Design review of the part shown in the three views and the two pictorial views. Dimensions are in mm from the part's minimum x, y and z. A direction names the side the tool comes from. Coordinates: 2 decimals unless noted, no trailing zeros. Write each loop counter-clockwise with the first axis right and the second up, starting at its lowest first coordinate (ties: lowest second). Pieces come first, ordered by that corner, then holes. Notation, with made-up numbers: (0, -2.75) -> (6, -2.75) arc R17 ccw to (6, 19.25) -> close; hole circle Ø5 at (73, -33). An arc over 180 degrees is marked (long way). Answer in a Markdown table with one row per item. Add a question column.
Item 1: Take a section at A-A, the plane x = 67. Write out the cut boundary in (y, z).
Item 2: To check wall thickness, follow line 1 (Y direction, x = 63, z = 36.5); line 2 (Z direction, x = 106, y = 40); line 3 (Z direction, x = 150, y = 5.5) (1 decimal). State the ranges of each line that lie inside material, in increasing order.
Item 3: Take a section at D-D, the plane x = 111. Write out the cut boundary in (y, z).
Item 4: For the marked faces 1 and 2, list the 3-axis set-ups (+Z, -Z, +X, -X, +Y, -Y) from which the entire face can be reached by the end or side of a thin tool; tool diameter is ignored.
Item 5: Take a section at B-B, the plane z = 10. Write out the cut boundary in (x, y), and give its area (3 significant figures).
Item 6: Clearance check with flat-ended pins moving along their axes: P1, Ø3.5, axis at y = 30, z = 51.5, coming from the +X side; P2, Ø16, axis at x = 91.5, z = 15, coming from the +Y side; P3, Ø12, axis at x = 81, y = 38, coming from the -Z side. State where each tip first meets the part, or that it passes through.
Item 7: Take a section at C-C, the plane y = 37. Write out the cut boundary in (x, z).
Item 8: Draft analysis for pull direction Z (two halves, no side actions). For the marked faces 3, 4 and 5, state which applies: released by +Z, released by -Z, zero draft, split by the parting line, or undercut.
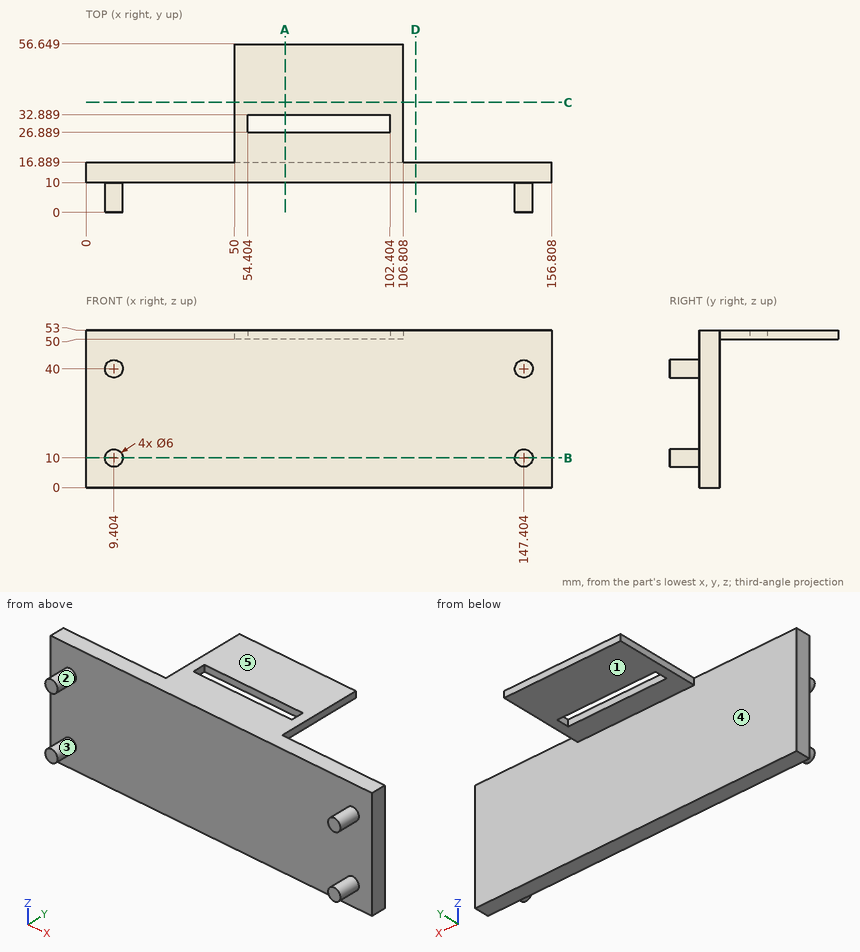
Answers:
| question | item | result |
|---|---|---|
| 1 | outline | (10, 0) -> (16.89, 0) -> (16.89, 50) -> (26.89, 50) -> (26.89, 53) -> (10, 53) -> close; (32.89, 50) -> (56.65, 50) -> (56.65, 53) -> (32.89, 53) -> close |
| 2 | line 1 | y = 10 to 16.89 |
| 2 | line 2 | z = 50 to 53 |
| 2 | line 3 | z = 8.5 to 11.5, 38.5 to 41.5 |
| 3 | outline | (10, 0) -> (16.89, 0) -> (16.89, 53) -> (10, 53) -> close |
| 4 | face 1 | -Z, +X, -X, +Y |
| 4 | face 2 | -Y |
| 5 | outline | (0, 10) -> (6.4, 10) -> (6.4, 0) -> (12.4, 0) -> (12.4, 10) -> (144.4, 10) -> (144.4, 0) -> (150.4, 0) -> (150.4, 10) -> (156.81, 10) -> (156.81, 16.89) -> (0, 16.89) -> close |
| 5 | area | 1,200 mm^2 |
| 6 | P1 | stops at x = 106.81 |
| 6 | P2 | stops at y = 16.89 |
| 6 | P3 | stops at z = 50 |
| 7 | outline | (50, 50) -> (106.81, 50) -> (106.81, 53) -> (50, 53) -> close |
| 8 | face 3 | undercut |
| 8 | face 4 | zero draft |
| 8 | face 5 | released by +Z |
